Model file for the job. Use its own axes, mm. Round coordinates to 2 decimals unless told otherwise and drop trailing zeros. Loops run counter-clockwise (first coordinate to the right, second up) from the corner with the lowest first, then second, coordinate; pieces in that order, holes last. Notation, with made-up numbers: (3.25, -20.5) - (26.25, -20.5) arc R26 ccw to (26.25, 3.5) - close; hole circle Ø7 at (-1.5, 47.25). An arc over 180 degrees is marked (long way). Answer as a JSON object with one key per item and string values.
from build123d import *

# Parameters (mm, degrees)
CUT_EXTRUDE1_DEPTH = 0.6
FILLET1_R          = 0.15


with BuildPart() as part:
    # Sketch4 → Revolve2 (revolve)
    with BuildSketch(Plane(origin=(0, 0, 0), x_dir=(0, 0, -1), z_dir=(1, 0, 0))):
        with BuildLine():
            Line((0, 0), (24, 0))
            Line((24, 0), (24, 0.95))
            Line((24, 0.95), (1.25, 0.95))
            Line((1.25, 0.95), (1.25, 1.63))
            ThreePointArc((1.25, 1.63), (0.348475184, 1.027058908), (0, 0))
        make_face()
    revolve(axis=Axis((0, 0, 0), (0, 0, -1)))

    # Sketch5 → Cut-Extrude1 (cut)
    with BuildSketch(Plane.XY):
        with BuildLine():
            Line((-0.375, -0.649519053), (-0.375, -1.87097888))
            Line((-0.375, -1.87097888), (0.375, -1.87097888))
            Line((0.375, -1.87097888), (0.375, -0.649519053))
            ThreePointArc((0.375, -0.649519053), (0.75, 0), (0.375, 0.649519053))
            Line((0.375, 0.649519053), (0.375, 1.87097888))
            Line((0.375, 1.87097888), (-0.375, 1.87097888))
            Line((-0.375, 1.87097888), (-0.375, 0.649519053))
            ThreePointArc((-0.375, 0.649519053), (-0.75, 0), (-0.375, -0.649519053))
        make_face()
    extrude(amount=-CUT_EXTRUDE1_DEPTH, mode=Mode.SUBTRACT)

    # Fillet1
    fillet1_edges = [part.edges().sort_by_distance(p)[0] for p in [
        (0, -1.63, -1.25),
        (0, -0.95, -24),
    ]]
    fillet(fillet1_edges, radius=FILLET1_R)


solid = part.part
1) Slice it at A-A on z = -20.5. List the corners of the cut face in (x, y).
Values follow:
{"outline": "circle Ø1.9 at (0, 0)"}
2) Drop flat-ended pins along their axis: P1, Ø1, axis at x = -0.5, z = -7, coming from the -Y side; P2, Ø1.5, axis at y = -0.5, z = -7, coming from the +X side; P3, Ø0.5, axis at y = 1, z = -0.5, coming from the -X side. Give the stop position or say it passes through.
Values follow:
{"P1": "y = -0.95", "P2": "x = 0.95", "P3": "x = -1.07"}
3) Two-plate mould, pull along Y, no slides. Class faces 1 (the flat face through (0, 0, -0.6)), 2 (the flat face through (0, 0, -24)), 3 (the cylindrical face through (0.04, -0.95, -12.39)): pulls with the +Y half, pulls with the -Y half, needs draft (parallel to the pull), parting line crosses it, or undercut.
Values follow:
{"face 1": "undercut", "face 2": "needs draft", "face 3": "parting line crosses it"}
4) Probe probe 1 along X at (y, z) = (-0.05, -12.5); probe 2 along Z at (x, y) = (0.05, 1); probe 3 along Z at (x, y) = (-0.7, 0.8). List the from-to ranges inside material, lowest first.
Values follow:
{"probe 1": "-0.95 to 0.95", "probe 2": "-1.25 to -0.6", "probe 3": "-1.25 to -0.38"}
